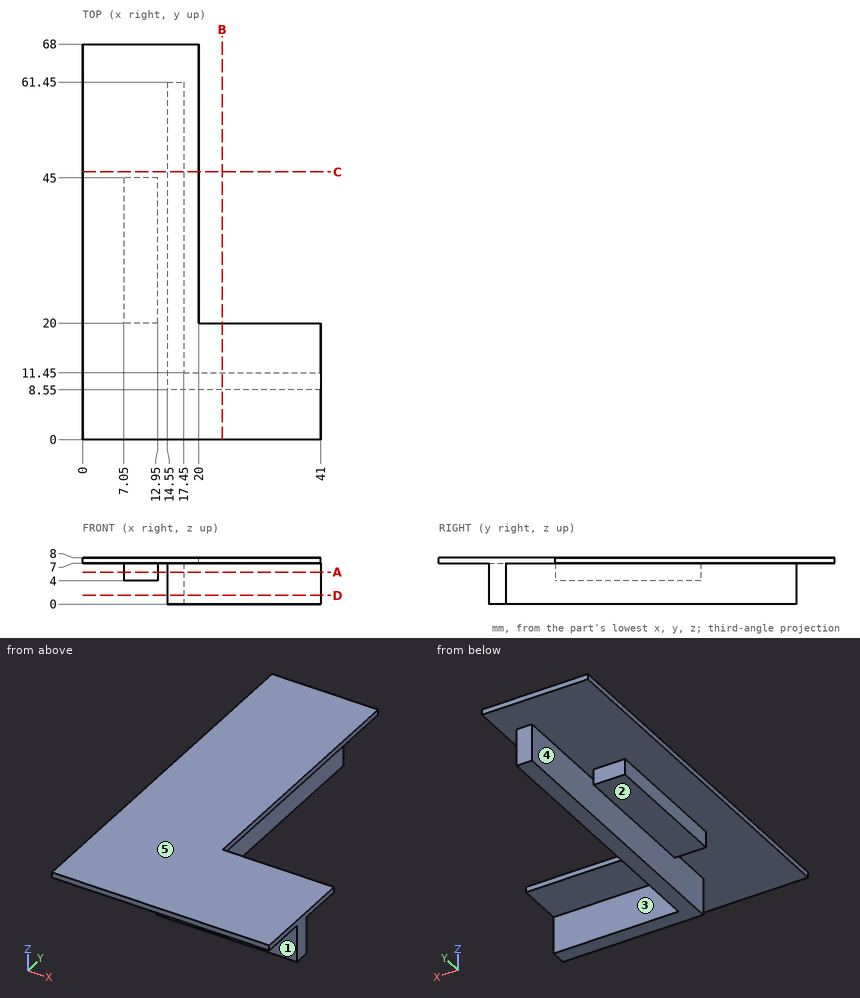
For this review, use the dimensioned drawing (mm, ordinates from the lowest corner) and the shaded views. A direction names the side the tool comes from. Coordinates: 2 decimals unless noted, no trailing zeros. Loops run counter-clockwise (first coordinate to the right, second up) from the corner with the lowest first, then second, coordinate; pieces in that order, holes last. Notation, with made-up numbers: (15, 9.5) -> (23, 9.5) arc R20 cw to (23, 24.5) -> close; hole circle Ø6 at (-31.75, -15). An arc over 180 degrees is marked (long way). Use a Markdown table: item, result. Add a question column.
1. Draft analysis for pull direction X (two halves, no side actions). For the marked faces 4 and 5, state which applies: pulls with the +X half, pulls with the -X half, needs draft (parallel to the pull), parting line crosses it, or undercut.
2. Add section D-D on z = 1.5. Write out the cut boundary in (x, y).
3. Add section C-C on y = 46. Write out the cut boundary in (x, z).
4. Machinability: for the marked faces 1, 2 and 3, which of the approach directions +Z, -Z, +X, -X, +Y, -Y give a long, thin tool a straight path to every point of the face, cutting with its end or side? Answer none if there is none.
5. Add section A-A on z = 5.5. Write out the cut boundary in (x, y).
6. Add section B-B on x = 24. Write out the cut boundary in (y, z).
7. Clearance check with flat-ended pins moving along their axes: pin 1 Ø0.9 at (x, z) = (16.5, 2.5) entering from +Y; pin 2 Ø4 at (y, z) = (22.5, 3.5) entering from +X; pin 3 Ø0.8 at (y, z) = (55, 7.5) entering from +X. State where each tip first meets the part, or that it passes through.
8. To check wall thickness, follow line 1 (X direction, y = 32, z = 4.75); line 2 (Y direction, x = 35.5, z = 4.75); line 3 (Z direction, x = 38.5, y = 13.5). State the ranges of each line that lie inside material, in increasing order.
Returned:
| question | item | result |
|---|---|---|
| 1 | face 4 | undercut |
| 1 | face 5 | needs draft |
| 2 | outline | (14.55, 8.55) -> (41, 8.55) -> (41, 11.45) -> (17.45, 11.45) -> (17.45, 61.45) -> (14.55, 61.45) -> close |
| 3 | outline | (0, 7) -> (14.55, 7) -> (14.55, 0) -> (17.45, 0) -> (17.45, 7) -> (20, 7) -> (20, 8) -> (0, 8) -> close |
| 4 | face 1 | -Z, +X, -X, -Y |
| 4 | face 2 | -Z, -X, +Y, -Y |
| 4 | face 3 | -Z, +X, +Y |
| 5 | outline | (7.05, 20) -> (12.95, 20) -> (12.95, 45) -> (7.05, 45) -> close; (14.55, 8.55) -> (41, 8.55) -> (41, 11.45) -> (17.45, 11.45) -> (17.45, 61.45) -> (14.55, 61.45) -> close |
| 6 | outline | (0, 7) -> (8.55, 7) -> (8.55, 0) -> (11.45, 0) -> (11.45, 7) -> (20, 7) -> (20, 8) -> (0, 8) -> close |
| 7 | pin 1 | stops at y = 61.45 |
| 7 | pin 2 | stops at x = 17.45 |
| 7 | pin 3 | stops at x = 20 |
| 8 | line 1 | x = 7.05 to 12.95, 14.55 to 17.45 |
| 8 | line 2 | y = 8.55 to 11.45 |
| 8 | line 3 | z = 7 to 8 |
